Geometry check sheet. Reference: the model listing, model coordinates, mm. Round coordinates to 2 decimals unless told otherwise and drop trailing zeros. Write each loop counter-clockwise with the first axis right and the second up, starting at its lowest first coordinate (ties: lowest second). Pieces come first, ordered by that corner, then holes. Notation, with made-up numbers: M -8.75,-32.5 L 8.25,-32.5 A27 ccw 8.25,-10.5 Z; hole C -34,-10 d5. An arc over 180 degrees is marked long. Put each result on its own line as item: value. Start each with the question number.
(1) Section check B-B on y = 11. Record the cut outline in (x, z), then the cut area to 3 significant figures.
(2) Material ranges on probe 1 along Y at (x, z) = (-12.5, 0.5); probe 2 along X at (y, z) = (0.5, 1.5); probe 3 along Y at (x, z) = (-17, 6.25), recorded low to high.
(3) Section check C-C on z = 2.25. Count the separate pieces of the cut face and the enclosed holes in it, then the cut area to 3 significant figures.
(4) Gauge pin test, flat end, axial feed: pin 1 (3.5 mm diameter, centred on x = 0.21, y = -12.91, fed in from -Z). Record the tip position at first contact, or that the pin passes through.
(5) Mould release check, pull along X, two halves, no side actions. Record for faces 1 (the cylindrical face through (22.87, -17.37, 3.22)), 2 (the flat face through (0, -27.5, 3)), 3 (the cylindrical face through (1.075, 25.107, 3.219)): pulls with the +X half, pulls with the -X half, needs draft (parallel to the pull), parting line crosses it, or undercut.
(6) Section check A-A on x = 0. Record the cut outline in (y, z).
from build123d import *

# Parameters (mm, degrees)
SKETCH1_W                 = 60
SKETCH1_H                 = 55
BOSS_EXTRUDE1_DEPTH       = 6.35
SKETCH2_R                 = 2
CUT_EXTRUDE1_DEPTH        = 6.35
SKETCH3_R                 = 3
CUT_EXTRUDE2_DEPTH        = 42.189470742
LPATTERN1_COUNT           = 3
LPATTERN1_PITCH           = 12.7
LPATTERN2_COUNT           = 3
LPATTERN2_PITCH           = 12.7
LPATTERN2_COPY_1_SKETCH_R = 3
LPATTERN2_COPY_1_DEPTH    = 42.189470742
LPATTERN2_COPY_2_SKETCH_R = 3
LPATTERN2_COPY_2_DEPTH    = 42.189470742
LPATTERN2_COPY_3_SKETCH_R = 3
LPATTERN2_COPY_3_DEPTH    = 42.189470742
LPATTERN2_COPY_4_SKETCH_R = 3
LPATTERN2_COPY_4_DEPTH    = 42.189470742


with BuildPart() as part:
    # Sketch1 → Boss-Extrude1 (new body)
    with BuildSketch(Plane.XY):
        Rectangle(SKETCH1_W, SKETCH1_H)
    extrude(amount=BOSS_EXTRUDE1_DEPTH)

    # Sketch2 → Cut-Extrude1 (cut)
    with BuildSketch(Plane.XY.offset(6.35)):
        with BuildLine():
            Line((-30, 27.5), (-30, 10))
            ThreePointArc((-30, 10), (-22.799858447, 17.492776255), (-20, 27.5))
            Line((-20, 27.5), (-30, 27.5))
        make_face()
        with BuildLine():
            ThreePointArc((-20, -27.5), (-22.799858447, -17.492776255), (-30, -10))
            Line((-30, -10), (-30, -27.5))
            Line((-30, -27.5), (-20, -27.5))
        make_face()
        with BuildLine():
            ThreePointArc((30, -10), (22.799858447, -17.492776255), (20, -27.5))
            Line((20, -27.5), (30, -27.5))
            Line((30, -27.5), (30, -10))
        make_face()
        with BuildLine():
            Line((30, 27.5), (20, 27.5))
            ThreePointArc((20, 27.5), (22.799858447, 17.492776255), (30, 10))
            Line((30, 10), (30, 27.5))
        make_face()
        with Locations((17.07106781, 17.07106781)):
            Circle(SKETCH2_R)
        with Locations((23.535533905, 0)):
            Circle(SKETCH2_R)
        with Locations((17.07106781, -17.07106781)):
            Circle(SKETCH2_R)
        with Locations((-17.07106781, -17.07106781)):
            Circle(SKETCH2_R)
        with Locations((-23.535533905, 0)):
            Circle(SKETCH2_R)
        with Locations((-17.07106781, 17.07106781)):
            Circle(SKETCH2_R)
        with Locations((0, -23.42106781)):
            Circle(SKETCH2_R)
        with Locations((0, 23.42106781)):
            Circle(SKETCH2_R)
    extrude(amount=-CUT_EXTRUDE1_DEPTH, mode=Mode.SUBTRACT)

    # Sketch3 → Cut-Extrude2 (cut, through all)
    with BuildSketch(Plane.XY.offset(6.35)):
        with Locations((-12.490915526, 12.490915526)):
            Circle(SKETCH3_R)
    cut_extrude2 = extrude(amount=-CUT_EXTRUDE2_DEPTH, mode=Mode.SUBTRACT)

    # LPattern1: Cut-Extrude2 ×3
    with Locations(*[(i * LPATTERN1_PITCH, 0, 0) for i in range(1, LPATTERN1_COUNT)]):
        add(cut_extrude2, mode=Mode.SUBTRACT)

    # LPattern2: Cut-Extrude2 ×3
    with Locations(*[(0, -i * LPATTERN2_PITCH, 0) for i in range(1, LPATTERN2_COUNT)]):
        add(cut_extrude2, mode=Mode.SUBTRACT)

    # LPattern2 copy 1 sketch → LPattern2 copy 1 (cut, through all)
    with BuildSketch(Plane(origin=(12.7, -12.7, 6.35), x_dir=(1, 0, 0), z_dir=(0, 0, 1))):
        with Locations((-12.490915526, 12.490915526)):
            Circle(LPATTERN2_COPY_1_SKETCH_R)
    extrude(amount=-LPATTERN2_COPY_1_DEPTH, mode=Mode.SUBTRACT)

    # LPattern2 copy 2 sketch → LPattern2 copy 2 (cut, through all)
    with BuildSketch(Plane(origin=(12.7, -25.4, 6.35), x_dir=(1, 0, 0), z_dir=(0, 0, 1))):
        with Locations((-12.490915526, 12.490915526)):
            Circle(LPATTERN2_COPY_2_SKETCH_R)
    extrude(amount=-LPATTERN2_COPY_2_DEPTH, mode=Mode.SUBTRACT)

    # LPattern2 copy 3 sketch → LPattern2 copy 3 (cut, through all)
    with BuildSketch(Plane(origin=(25.4, -12.7, 6.35), x_dir=(1, 0, 0), z_dir=(0, 0, 1))):
        with Locations((-12.490915526, 12.490915526)):
            Circle(LPATTERN2_COPY_3_SKETCH_R)
    extrude(amount=-LPATTERN2_COPY_3_DEPTH, mode=Mode.SUBTRACT)

    # LPattern2 copy 4 sketch → LPattern2 copy 4 (cut, through all)
    with BuildSketch(Plane(origin=(25.4, -25.4, 6.35), x_dir=(1, 0, 0), z_dir=(0, 0, 1))):
        with Locations((-12.490915526, 12.490915526)):
            Circle(LPATTERN2_COPY_4_SKETCH_R)
    extrude(amount=-LPATTERN2_COPY_4_DEPTH, mode=Mode.SUBTRACT)


solid = part.part
Answers follow:
1. outline: M -28.54,0 L -15.09,0 L -15.09,6.35 L -28.54,6.35 Z; M -9.89,0 L -2.39,0 L -2.39,6.35 L -9.89,6.35 Z; M 2.81,0 L 10.31,0 L 10.31,6.35 L 2.81,6.35 Z; M 15.51,0 L 28.54,0 L 28.54,6.35 L 15.51,6.35 Z
1. area: 263 mm^2
2. probe 1: y = -27.5 to -15.91, -9.91 to -3.21, 2.79 to 9.49, 15.49 to 27.5
2. probe 2: x = -30 to -25.47, -21.6 to -15.41, -9.58 to -2.71, 3.12 to 9.99, 15.82 to 21.6, 25.47 to 30
2. probe 3: y = -27.5 to -19.07, -15.07 to 15.07, 19.07 to 27.5
3. separate pieces: 1
3. enclosed holes: 17
3. area: 2,460 mm^2
4. pin 1: passes through
5. face 1: pulls with the +X half
5. face 2: needs draft
5. face 3: undercut
6. outline: M -27.5,0 L -25.42,0 L -25.42,6.35 L -27.5,6.35 Z; M -21.42,0 L -15.9,0 L -15.9,6.35 L -21.42,6.35 Z; M -9.92,0 L -3.2,0 L -3.2,6.35 L -9.92,6.35 Z; M 2.78,0 L 9.5,0 L 9.5,6.35 L 2.78,6.35 Z; M 15.48,0 L 21.42,0 L 21.42,6.35 L 15.48,6.35 Z; M 25.42,0 L 27.5,0 L 27.5,6.35 L 25.42,6.35 Z
